Geometry: final body of the model. Coordinates: model frame, mm. Coordinates: 2 decimals unless noted, no trailing zeros. Loops run counter-clockwise (first coordinate to the right, second up) from the corner with the lowest first, then second, coordinate; pieces in that order, holes last. Notation, with made-up numbers: (44, 75) - (73, 75) arc R13 cw to (73, 80) - close; hole circle Ø4 at (61.5, 8). An arc over 180 degrees is marked (long way). Write each question's results on one line, items separated by ' | '. Start each with the question number.
from build123d import *

# Parameters (mm, degrees)
BOSS_EXTRU_1_DEPTH      = 6.35
ENL_V_MAT_EXTRU_1_REACH = 84.663
ESQUISSE3_R             = 1.5
ENL_V_MAT_EXTRU_2_DEPTH = 6.35


with BuildPart() as part:
    # Esquisse1 → Boss.-Extru.1 (new body)
    with BuildSketch(Plane.XY):
        with BuildLine():
            Line((0, 6), (76.2, 6))
            ThreePointArc((76.2, 6), (82.2, 0), (76.2, -6))
            Line((76.2, -6), (0, -6))
            ThreePointArc((0, -6), (-6, 0), (0, 6))
        make_face()
    extrude(amount=BOSS_EXTRU_1_DEPTH)

    # Esquisse2 → Enlèv. mat.-Extru.1 (cut, up to next)
    with BuildSketch(Plane.XY.offset(6.35), mode=Mode.PRIVATE) as enl_v_mat_extru_1_sk1:
        with BuildLine():
            Line((-2.214723459, -2.275), (2.214723459, -2.275))
            ThreePointArc((2.214723459, -2.275), (0, 3.175), (-2.214723459, -2.275))
        make_face()
    enl_v_mat_extru_1_tool1 = extrude(enl_v_mat_extru_1_sk1.sketch, amount=-ENL_V_MAT_EXTRU_1_REACH, mode=Mode.PRIVATE) & part.part
    add(enl_v_mat_extru_1_tool1.solids().sort_by_distance((0, 0.25037, 6.35))[0], mode=Mode.SUBTRACT)

    # Esquisse3 → Enlèv. mat.-Extru.2 (cut)
    with BuildSketch(Plane.XY.offset(6.35)):
        with Locations((76.2, 0)):
            Circle(ESQUISSE3_R)
    extrude(amount=-ENL_V_MAT_EXTRU_2_DEPTH, mode=Mode.SUBTRACT)


solid = part.part
1) Section query C-C on y = -4. Output: boundary loops of the cut face in (x, z), and give its area (3 significant figures).
2) Pull-direction query (Y, two-part tool) for faces 1 (the flat face through (39, -6, 3)), 2 (the flat face through (39, 0, 6.35)), 3 (the cylindrical face through (0.105, 3.173, 3.219)), 4 (the flat face through (0, -2.275, 3)); classes: released by +Y, released by -Y, zero draft, split by the parting line, or undercut.
3) Material intervals for line 1 (X direction, y = 0.25, z = 5.5); line 2 (Y direction, x = 76.2, z = 4); line 3 (Y direction, x = 0, z = 3) (3 decimals), sorted ascending. Write a range as [from, to].
4) Section query B-B on z = 5.25. Output: boundary loops of the cut face in (x, y) (3 decimals), and give its area (3 significant figures).
5) Section query A-A on y = 0. Output: boundary loops of the cut face in (x, z) (3 decimals), and give its area (3 significant figures).
6) Pin query (flat end, axial travel): pin 1 Ø2.5 at (x, y) = (76.2, 0) entering from -Z; pin 2 Ø1.5 at (y, z) = (-1.5, 3.5) entering from -X. Return the tip coordinate at first contact, or that it passes through.
Returned:
1) outline: (-4.47, 0) - (80.67, 0) - (80.67, 6.35) - (-4.47, 6.35) - close | area: 541 mm²
2) face 1: released by -Y | face 2: zero draft | face 3: undercut | face 4: undercut
3) line 1: x = [-5.99, -3.17], [3.17, 74.72], [77.68, 82.19] | line 2: y = [-6, -1.5], [1.5, 6] | line 3: y = [-6, -2.275], [3.175, 6]
4) outline: (0, -6) - (76.2, -6) arc R6 ccw to (76.2, 6) - (0, 6) arc R6 ccw to start; hole (-2.215, -2.275) - (2.215, -2.275) arc R3.175 ccw (long way) to start; hole circle Ø3 at (76.2, 0) | area: 992 mm²
5) outline: (-6, 0) - (-3.175, 0) - (-3.175, 6.35) - (-6, 6.35) - close; (3.175, 0) - (74.7, 0) - (74.7, 6.35) - (3.175, 6.35) - close; (77.7, 0) - (82.2, 0) - (82.2, 6.35) - (77.7, 6.35) - close | area: 501 mm²
6) pin 1: passes through | pin 2: stops at x = -5.95
